Autodesk Inventor part; units mm, degrees
ref_plane "YZ Plane" through (0, 0, 0) normal (1, 0, 0) x (0, 1, 0)
ref_plane "XZ Plane" through (0, 0, 0) normal (0, 1, 0) x (-1, 0, 0)
ref_plane "XY Plane" through (0, 0, 0) normal (0, 0, 1) x (1, 0, 0)
sketch "Sketch2" plane through (0, 0, 0) normal (0, 0, 1) x (1, 0, 0)
  line L0 (-196.3166, 196.3166) -> (0, 277.6336)
  line L1 (0, 277.6336) -> (196.3166, 196.3166)
  line L2 (196.3166, 196.3166) -> (277.6336, 0)
  line L3 (277.6336, 0) -> (196.3166, -196.3166)
  line L4 (196.3166, -196.3166) -> (0, -277.6336)
  line L5 (0, -277.6336) -> (-196.3166, -196.3166)
  line L6 (-196.3166, -196.3166) -> (-277.6336, 0)
  line L7 (-277.6336, 0) -> (-196.3166, 196.3166)
  circle A0 centre (0, 0) radius 125
  dimension "d23" = 513
  dimension "d26" = 250
extrude "Plate1" add sketch "Sketch2" against normal blind 3
sketch "Sketch4" plane through (0, 0, 0) normal (0, 0, 1) x (1, 0, 0)
  circle A0 centre (0, 145) radius 6.25
  circle A1 centre (0, 0) radius 125
  dimension "d16" = 12.5
  dimension "d17" = 145
extrude "Extrusion1" cut sketch "Sketch4" against normal up to surface (3 mm away) contours A0
pattern_circular "Circular Pattern1" count 8 over 360 about axis through (0, 0, -10) along (0, 0, 1) of "Extrusion1"
equation "\"d23\" = Барабан_габарит_по_кассетам"
equation "\"d26\" = Вал_ось_диаметр_НОС"
equation "\"d15\" = Thickness"
equation "\"BendRadius\" = Thickness"
equation "\"BendReliefWidth\" = Thickness"
equation "\"BendReliefDepth\" = 0.5 * Thickness"
equation "\"CornerReliefSize\" = 4 * Thickness"
equation "\"MinimumRemnant\" = 2 * Thickness"
equation "\"TransitionRadius\" = BendRadius"
equation "\"JacobiRadiusSize\" = BendRadius"
equation "\"GapSize\" = Thickness"
properties part number "DMF 01 21 cylinder butt end nose"
For this review, take the finished solid that the model builds, in its own axes (mm). Coordinates: 2 decimals unless noted, no trailing zeros. Loops run counter-clockwise (first coordinate to the right, second up) from the corner with the lowest first, then second, coordinate; pieces in that order, holes last. Notation, with made-up numbers: (-21, 63.25) -> (10, 63.25) arc R14 cw to (10, 79.25) -> close; hole circle Ø2 at (89.5, 62). An arc over 180 degrees is marked (long way). Write each question's results on one line, items separated by ' | '.
Q1. Add section A-A, the plane z = -1.85. Count the separate pieces of the cut face and the enclosed holes in it, then the cut area to 3 significant figures.
Taken from the geometry:
separate pieces: 1 | enclosed holes: 9 | area: 168,000 mm²
Q2. For pin 1 Ø1 at (x, z) = (171, -2.5) entering from -Y, flat-tipped, find the tip position at first contact; note if it passes through.
Taken from the geometry:
pin 1: y = -207.01
Q3. Add section C-C, the plane y = 174. State the section outline as (x, z) points, then the cut area to 3 significant figures.
Taken from the geometry:
outline: (-205.56, -3) -> (205.56, -3) -> (205.56, 0) -> (-205.56, 0) -> close | area: 1,230 mm²
Q4. To check wall thickness, follow line 1 along Y through (x, z) = (0, -2.3); line 2 along X through (y, z) = (-79, -1.1); line 3 along Y through (x, z) = (-149.5, -1). State the ranges of each line that lie inside material, in increasing order. Write a range as [from, to].
Taken from the geometry:
line 1: [-277.63, -151.25], [-138.75, -125], [125, 138.75], [151.25, 277.63] | line 2: [-244.91, -96.87], [96.87, 244.91] | line 3: [-215.71, -4.34], [4.34, 215.71]
Q5. Mouldability with a two-part tool opening along Y and no side actions: class faces 1 (the flat face through (96.784, 237.544, -1.479)), 2 (the cylindrical face through (139.455, -2.884, -1.479)), 3 (the flat face through (-127, 4, -3)) as +Y half, -Y half, draft (parallel to the pull), parting line (faces both ways), or undercut.
Taken from the geometry:
face 1: +Y half | face 2: undercut | face 3: draft
Q6. Add section D-D, the plane x = 172. State the section outline as (y, z) points.
Taken from the geometry:
outline: (-206.39, -3) -> (206.39, -3) -> (206.39, 0) -> (-206.39, 0) -> close
Q7. Add section B-B, the plane y = 20. State the section outline as (x, z) points, then the cut area to 3 significant figures.
Taken from the geometry:
outline: (-269.35, -3) -> (-123.39, -3) -> (-123.39, 0) -> (-269.35, 0) -> close; (123.39, -3) -> (269.35, -3) -> (269.35, 0) -> (123.39, 0) -> close | area: 876 mm²
